Verification items for the finished model (mm, model axes). A direction names the side the tool comes from. Coordinates: 2 decimals unless noted, no trailing zeros. Order: outer loops, then holes, each group sorted by start corner. A loop starts at its lowest first (then second) coordinate and runs counter-clockwise, first axis right, second up. Notation, with made-up numbers: (-5, 18.5) - (42, 18.5) arc R24 cw to (42, 40.5) - close; hole circle Ø8 at (-11.75, 9.25). An arc over 180 degrees is marked (long way). Answer as CSV lines item,"result". Start each with the question number.
1. Section check B-B (z = 0). Record the cut outline in (x, y).
2. Material ranges on L1, parallel to X at y = 19.35, z = 0; L2, parallel to X at y = 13.75, z = 0; L3, parallel to Y at x = -0.25, z = 13.75, recorded low to high. Write a range as [from, to].
3. Go/stop test with flat-tipped pins: pin 1 (3 mm diameter, centred on y = 18, z = -4, fed in from +X); pin 2 (3 mm diameter, centred on y = 9.5, z = 2, fed in from +X); pin 3 (2 mm diameter, centred on x = 1.5, y = 12.5, fed in from -Z). Record where each tip stops, or that it passes through.
4. Section check A-A (y = 20). Record the cut outline in (x, z).
5. Section check C-C (x = 11.5). Record the cut outline in (y, z).
6. Mould release check, pull along X, two halves, no side actions. Record for faces 1 (the cylindrical face through (-7.493, 7.888, -0.33)), 2 (the flat face through (3, 0, 3)), 3 (the cylindrical face through (9.5, 18.79, -0.07)): pulls with the +X half, pulls with the -X half, needs draft (parallel to the pull), parting line crosses it, or undercut.
7. Section check D-D (x = -1). Record the cut outline in (y, z).
8. Set-up check for faces 4 (the cylindrical face through (6.691, 18.712, 12.864)), 5 (the flat face through (6, 16, 6)): record each of +Z, -Z, +X, -X, +Y, -Y from which the full face is reachable in a straight line by a thin tool's end or side.
from build123d import *

# Parameters (mm, degrees)
SKETCH1_R           = 7.5
SKETCH1_R_2         = 4
BOSS_EXTRUDE1_DEPTH = 16
SKETCH2_R           = 14.5
SKETCH2_R_2         = 7.5
BOSS_EXTRUDE2_DEPTH = 5.5
SKETCH3_R           = 7.5
SKETCH3_R_2         = 4
BOSS_EXTRUDE3_DEPTH = 5.5
SKETCH4_R           = 1.5
CUT_EXTRUDE1_DEPTH  = 5.5


with BuildPart() as part:
    # Sketch1 → Boss-Extrude1 (new body)
    with BuildSketch(Plane(origin=(0, 0, 0), x_dir=(1, 0, 0), z_dir=(0, 1, 0))):
        Circle(SKETCH1_R)
        Circle(SKETCH1_R_2, mode=Mode.SUBTRACT)
    extrude(amount=BOSS_EXTRUDE1_DEPTH)



with BuildPart() as body_2:
    # Sketch2 → Boss-Extrude2 (new body)
    with BuildSketch(Plane(origin=(0, 16, 0), x_dir=(1, 0, 0), z_dir=(0, 1, 0))):
        Circle(SKETCH2_R)
        Circle(SKETCH2_R_2, mode=Mode.SUBTRACT)
    extrude(amount=BOSS_EXTRUDE2_DEPTH)


with BuildPart() as part_1:
    add(part.part)

    add(body_2.part)  # Boss-Extrude3 merges body 2
    # Sketch3 → Boss-Extrude3 (add)
    with BuildSketch(Plane(origin=(0, 16, 0), x_dir=(1, 0, 0), z_dir=(0, 1, 0))):
        Circle(SKETCH3_R)
        Circle(SKETCH3_R_2, mode=Mode.SUBTRACT)
    extrude(amount=BOSS_EXTRUDE3_DEPTH)

    # Sketch4 → Cut-Extrude1 (cut)
    with BuildSketch(Plane(origin=(0, 21.5, 0), x_dir=(1, 0, 0), z_dir=(0, 1, 0))):
        with Locations((11, 0)):
            Circle(SKETCH4_R)
        with BuildLine():
            ThreePointArc((1.5, -11), (1.060660172, -9.939339828), (0, -9.5))
            Line((0, -9.5), (0, -12.5))
            ThreePointArc((0, -12.5), (1.060660172, -12.060660172), (1.5, -11))
        make_face()
        with BuildLine():
            Line((0, -12.5), (0, -9.5))
            ThreePointArc((0, -9.5), (-1.5, -11), (0, -12.5))
        make_face()
        with Locations((-11, 0)):
            Circle(SKETCH4_R)
        with BuildLine():
            ThreePointArc((1.5, 11), (1.060660172, 12.060660172), (0, 12.5))
            Line((0, 12.5), (0, 9.5))
            ThreePointArc((0, 9.5), (1.060660172, 9.939339828), (1.5, 11))
        make_face()
        with BuildLine():
            Line((0, 9.5), (0, 12.5))
            ThreePointArc((0, 12.5), (-1.5, 11), (0, 9.5))
        make_face()
    extrude(amount=-CUT_EXTRUDE1_DEPTH, mode=Mode.SUBTRACT)


solid = part_1.part
Evaluation:
1,outline,"(-14.5, 16) - (-12.5, 16) - (-12.5, 21.5) - (-14.5, 21.5) - close; (-9.5, 16) - (-7.5, 16) - (-7.5, 0) - (-4, 0) - (-4, 21.5) - (-9.5, 21.5) - close; (4, 0) - (7.5, 0) - (7.5, 16) - (9.5, 16) - (9.5, 21.5) - (4, 21.5) - close; (12.5, 16) - (14.5, 16) - (14.5, 21.5) - (12.5, 21.5) - close"
2,L1,"x = [-14.5, -12.5], [-9.5, -4], [4, 9.5], [12.5, 14.5]"
2,L2,"x = [-7.5, -4], [4, 7.5]"
2,L3,"y = [16, 21.5]"
3,pin 1,"stops at x = 14.28"
3,pin 2,"stops at x = 7.48"
3,pin 3,"stops at z = -7.48"
4,outline,"circle Ø29 at (0, 0); hole circle Ø3 at (-11, 0); hole circle Ø8 at (0, 0); hole circle Ø3 at (0, -11); hole circle Ø3 at (0, 11); hole circle Ø3 at (11, 0)"
5,outline,"(16, -8.83) - (21.5, -8.83) - (21.5, -1.41) - (16, -1.41) - close; (16, 1.41) - (21.5, 1.41) - (21.5, 8.83) - (16, 8.83) - close"
6,face 1,"parting line crosses it"
6,face 2,"needs draft"
6,face 3,"undercut"
7,outline,"(0, -7.43) - (16, -7.43) - (16, -9.88) - (21.5, -9.88) - (21.5, -3.87) - (0, -3.87) - close; (0, 3.87) - (21.5, 3.87) - (21.5, 9.88) - (16, 9.88) - (16, 7.43) - (0, 7.43) - close; (16, -14.47) - (21.5, -14.47) - (21.5, -12.12) - (16, -12.12) - close; (16, 12.12) - (21.5, 12.12) - (21.5, 14.47) - (16, 14.47) - close"
8,face 4,"+Y, -Y"
8,face 5,"-Y"
